Autodesk Inventor part; units mm, degrees
ref_plane "YZ Plane" through (0, 0, 0) normal (1, 0, 0) x (0, 1, 0)
ref_plane "XZ Plane" through (0, 0, 0) normal (0, 1, 0) x (-1, 0, 0)
ref_plane "XY Plane" through (0, 0, 0) normal (0, 0, 1) x (1, 0, 0)
sketch "Sketch2" plane through (0, 0, 0) normal (0, 0, 1) x (1, 0, 0)
  line L0 (-47.5, 20) -> (47.5, 20)
  line L1 (47.5, 20) -> (47.5, -25)
  line L2 (47.5, -25) -> (-47.5, -25)
  line L3 (-47.5, -25) -> (-47.5, 20)
  line L4 (-52.5, 20) -> (52.5, 20)
  line L5 (52.5, 20) -> (52.5, -25)
  line L6 (52.5, -25) -> (-52.5, -25)
  line L7 (-52.5, -25) -> (-52.5, 20)
  line L8 (-47.5, 15) -> (47.5, 15)
  line L9 (47.5, 15) -> (47.5, -20)
  line L10 (47.5, -20) -> (-47.5, -20)
  line L11 (-47.5, -20) -> (-47.5, 15)
  point P0 (0, 0)
  dimension "d4" = 95
  dimension "d5" = 45
  dimension "d6" = 47.5
  dimension "d7" = 20
  dimension "d8" = 5
  dimension "d9" = 5
  dimension "d10" = 5
  dimension "d11" = 5
  dimension "d12" = 45
  dimension "d13" = 5
extrude "Extrusion1" add sketch "Sketch2" against normal blind 210 contours L0 L1 L8 L3 | L3 L6 L7 L4 | L4 L5 L6 L1 | L10 L1 L2 L3
sketch "Sketch3" plane through (0, 0, -210) normal (0, 0, -1) x (-1, 0, 0)
  point P0 (0, 0)
sketch "Sketch4" plane through (0, 0, -210) normal (0, 0, -1) x (-1, 0, 0)
  line L0 (-52.5, -25) -> (-52.5, 20)
  line L1 (52.5, -25) -> (-52.5, -25)
  line L2 (-52.5, 20) -> (52.5, 20)
  line L3 (52.5, 20) -> (52.5, -25)
  line L4 (52.5, -25) -> (-52.5, -25)
  line L5 (-52.5, -25) -> (-52.5, 20)
  point P0 (0, 0)
extrude "Extrusion2" add sketch "Sketch4" along normal blind 5
sketch "Sketch8" plane through (-52.5, 20, -215) normal (0, 1, 0) x (1, 0, 0)
  line L0 (5, -215) -> (5, -5)
  line L1 (5, -5) -> (15, -5)
  line L2 (15, -5) -> (15, -210)
  line L3 (15, -210) -> (5, -210)
  line L4 (5, -210) -> (5, -5)
  line L5 (100, -215) -> (100, -5)
  line L6 (100, -5) -> (90, -5)
  line L7 (90, -5) -> (90, -210)
  line L8 (90, -210) -> (100, -210)
  line L9 (100, -210) -> (100, -5)
  point P0 (52.5, -215)
  point P1 (100, -210)
  dimension "d33" = 10
  dimension "d34" = 205
  dimension "d35" = 10
extrude "Extrusion6" cut sketch "Sketch8" against normal blind 5
sketch "Sketch11" plane through (-52.5, -25, 0) normal (0, -1, 0) x (1, 0, 0)
  line L0 (0, 0) -> (0, -215)
  line L1 (0, 0) -> (105, 0)
  line L2 (105, 0) -> (105, 5)
  line L3 (105, 5) -> (0, 5)
  line L4 (0, 5) -> (0, 0)
  line L5 (0, 0) -> (105, 0)
  line L6 (0, 0) -> (3, 0)
  line L7 (3, 0) -> (3, 5)
  line L8 (3, 5) -> (0, 5)
  line L9 (0, 5) -> (0, 0)
  line L10 (105, 0) -> (102, 0)
  line L11 (102, 0) -> (102, 5)
  line L12 (102, 5) -> (105, 5)
  line L13 (105, 5) -> (105, 0)
  point P0 (52.5, 0)
  point P1 (3, 0)
  dimension "d48" = 5
  dimension "d49" = 3
  dimension "d50" = 3
extrude "Extrusion9" add sketch "Sketch11" against normal blind 5 contours L7 L3 L11 L1
extrude "Extrusion10" add sketch "Sketch11" against normal blind 45 contours L4 L3 L7 L1 | L11 L3 L2 L1
properties part number "Team29_PiBox"
Input: part model. Units: mm. Frame: model coordinates. A direction names the side the tool comes from. Give positions to 0.01 mm unless a question says otherwise; leave off trailing zeros. Loops run counter-clockwise (first coordinate to the right, second up) from the corner with the lowest first, then second, coordinate; pieces in that order, holes last. Notation, with made-up numbers: (-37.5, 78.5) -> (-13.5, 78.5) arc R17 ccw to (-13.5, 92.5) -> close; hole circle Ø7 at (62, 29.5). An arc over 180 degrees is marked (long way). Answer as a JSON object with one key per item and string values. Group by question number.
Item 1: Line query: probe 1 along X at (y, z) = (-12.5, -14.5); probe 2 along Y at (x, z) = (7.5, -185.5); probe 3 along X at (y, z) = (17, -195). Output: solid intervals per line, ascending.
Item 2: Pin query (flat end, axial travel): P1, Ø8, axis at x = -32.5, y = 1.5, coming from the +Z side. Return the tip coordinate at first contact, or that it passes through.
Item 3: Cut plane B-B, the plane x = 45. Return the cut outline in (y, z).
Item 4: Cut plane C-C, the plane y = 7.5. Return the cut outline in (x, z).
Item 5: Cut plane D-D, the plane x = -3. Return the cut outline in (y, z), and give its area (3 significant figures).
Item 6: Reachability of faces 1 (the flat face through (-49.5, 0, 2)), 2 (the flat face through (-1, -20, -101)), 3 (the flat face through (-37.5, 18, -109)) from +Z, -Z, +X, -X, +Y, -Y: full face, straight path, thin tool, end or side. Return the list, or none.
Item 7: Pull-direction query (Y, two-part tool) for faces 4 (the flat face through (-1, 15, -104)), 5 (the flat face through (42, 18, -5)), 6 (the flat face through (1, 20, -103)); classes: released by +Y, released by -Y, zero draft, split by the parting line, or undercut.
Item 8: Cut plane A-A, the plane z = -21. Return the cut outline in (x, y).
Checks:
{
 "1": {"probe 1": "x = -52.5 to -47.5, 47.5 to 52.5", "probe 2": "y = -25 to -20, 15 to 20", "probe 3": "x = -52.5 to -47.5, -37.5 to 37.5, 47.5 to 52.5"},
 "2": {"P1": "stops at z = -210"},
 "3": {"outline": "(-25, -215) -> (20, -215) -> (20, -210) -> (-20, -210) -> (-20, 5) -> (-25, 5) -> close; (15, -5) -> (20, -5) -> (20, 0) -> (15, 0) -> close"},
 "4": {"outline": "(-52.5, -215) -> (52.5, -215) -> (52.5, 5) -> (49.5, 5) -> (49.5, 0) -> (47.5, 0) -> (47.5, -210) -> (-47.5, -210) -> (-47.5, 0) -> (-49.5, 0) -> (-49.5, 5) -> (-52.5, 5) -> close"},
 "5": {"outline": "(-25, -215) -> (20, -215) -> (20, 0) -> (15, 0) -> (15, -210) -> (-20, -210) -> (-20, 5) -> (-25, 5) -> close", "area": "2,350 mm²"},
 "6": {"face 1": "+Z, +Y", "face 2": "+Z", "face 3": "+Y"},
 "7": {"face 4": "undercut", "face 5": "zero draft", "face 6": "released by +Y"},
 "8": {"outline": "(-52.5, -25) -> (52.5, -25) -> (52.5, 20) -> (47.5, 20) -> (47.5, -20) -> (-47.5, -20) -> (-47.5, 20) -> (-52.5, 20) -> close; (-37.5, 15) -> (37.5, 15) -> (37.5, 20) -> (-37.5, 20) -> close"}
}
